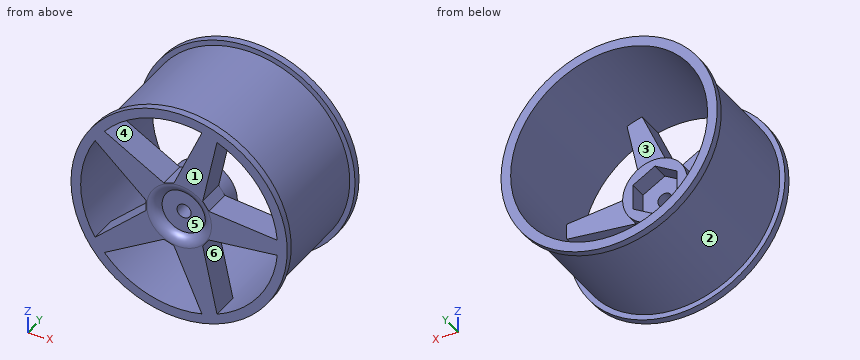
Autodesk Inventor part; units mm, degrees
ref_plane "YZ Plane" through (0, 0, 0) normal (1, 0, 0) x (0, 1, 0)
ref_plane "XZ Plane" through (0, 0, 0) normal (0, 1, 0) x (-1, 0, 0)
ref_plane "XY Plane" through (0, 0, 0) normal (0, 0, 1) x (1, 0, 0)
sketch "Sketch4" plane through (0, 0, 0) normal (0, 1, 0) x (-1, 0, 0)
  circle A0 centre (87.8745, -116.8332) radius 29.25
  point P0 (0, 0)
  dimension "d11" = 58.5
extrude "Extrusion4" add sketch "Sketch4" along normal blind 36
sketch "Sketch6" plane through (-87.8745, 0, -116.8332) normal (0, -1, 0) x (1, 0, 0)
  circle A0 centre (0, 0) radius 30.75
  point P0 (87.8745, 116.8332)
  dimension "d20" = 61.5
extrude "Extrusion6" add sketch "Sketch6" against normal blind 2
sketch "Sketch7" plane through (-87.8745, 36, -116.8332) normal (0, 1, 0) x (1, 0, 0)
  circle A0 centre (0, 0) radius 30.75
  point P0 (87.8745, -116.8332)
  dimension "d23" = 61.5
extrude "Extrusion7" add sketch "Sketch7" against normal blind 2
sketch "Sketch5" plane through (-87.8745, 0, -116.8332) normal (0, -1, 0) x (1, 0, 0)
  circle A0 centre (0, 0) radius 28
  circle A1 centre (0, 0) radius 29.25
  point P0 (87.8745, 116.8332)
  dimension "d16" = 0
  dimension "d17" = 0
  dimension "d26" = 56
extrude "Extrusion5" cut sketch "Sketch5" against normal blind 36 contours A0
sketch "Sketch8" plane through (-87.8745, 0, -116.8332) normal (0, -1, 0) x (1, 0, 0)
  circle A0 centre (0, 0) radius 8.5
  circle A1 centre (0, 0) radius 28
  line L0 (28, 0) -> (28, 2.25)
  line L1 (28, 0) -> (28, -2.25)
  line L2 (8.5, 0) -> (8.5, 4.3)
  line L3 (8.5, 0) -> (8.5, -4.3)
  line L4 (8.5, 4.3) -> (28, 2.25)
  line L5 (8.5, -4.3) -> (28, -2.25)
  arc A2 (27.9087, -2.2596) -> (27.9087, 2.2596) centre (0, 0) ccw
  line L6 (-1.4629, 9.4128) -> (6.5126, 27.3249)
  line L7 (2.6266, 8.084) -> (-1.4629, 9.4128)
  line L8 (2.6266, 8.084) -> (6.7162, 6.7552)
  line L9 (6.7162, 6.7552) -> (10.7924, 25.9343)
  arc A3 (10.7733, 25.8445) -> (6.4752, 27.241) centre (0, 0) ccw
  line L10 (-9.4041, 1.5174) -> (-23.975, 14.6377)
  line L11 (-6.8766, 4.9962) -> (-9.4041, 1.5174)
  line L12 (-6.8766, 4.9962) -> (-4.3492, 8.4749)
  line L13 (-4.3492, 8.4749) -> (-21.33, 18.2783)
  arc A4 (-21.2504, 18.2324) -> (-23.9068, 14.5763) centre (0, 0) ccw
  line L14 (-4.3492, -8.4749) -> (-21.33, -18.2783)
  line L15 (-6.8766, -4.9962) -> (-4.3492, -8.4749)
  line L16 (-6.8766, -4.9962) -> (-9.4041, -1.5174)
  line L17 (-9.4041, -1.5174) -> (-23.975, -14.6377)
  arc A5 (-23.9068, -14.5763) -> (-21.2504, -18.2324) centre (0, 0) ccw
  line L18 (6.7162, -6.7552) -> (10.7924, -25.9343)
  line L19 (2.6266, -8.084) -> (6.7162, -6.7552)
  line L20 (2.6266, -8.084) -> (-1.4629, -9.4128)
  line L21 (-1.4629, -9.4128) -> (6.5126, -27.3249)
  arc A6 (6.4752, -27.241) -> (10.7733, -25.8445) centre (0, 0) ccw
  line L22 (-1.4629, 9.4128) -> (-4.3492, 8.4749)
  line L23 (-9.4041, 1.5174) -> (-9.4041, -1.5174)
  line L24 (-4.3492, -8.4749) -> (-1.4629, -9.4128)
  line L25 (6.7162, -6.7552) -> (8.5, -4.3)
  line L26 (8.5, 4.3) -> (6.7162, 6.7552)
  line L27 (6.7162, 6.7552) -> (-1.4629, 9.4128)
  line L28 (-4.3492, 8.4749) -> (-9.4041, 1.5174)
  line L29 (-9.4041, -1.5174) -> (-4.3492, -8.4749)
  line L30 (-1.4629, -9.4128) -> (6.7162, -6.7552)
  line L31 (8.5, -4.3) -> (8.5, 4.3)
  point P0 (87.8745, 116.8332)
  point P1 (8.6525, 26.6296)
  point P2 (-22.6525, 16.458)
  point P3 (-22.6525, -16.458)
  point P4 (8.6525, -26.6296)
  dimension "d27" = 17
  dimension "d29" = 2.25
  dimension "d30" = 2.25
  dimension "d31" = 4.3
  dimension "d32" = 4.3
  dimension "d35" = 360
extrude "Extrusion8" add sketch "Sketch8" against normal blind 8 contours A0 | L3 L25 L19 A0 | A0 L8 L26 L2 | L2 L4 A1 L5 L3 | A0 L12 L22 L7 | L7 L6 A1 L9 L8 | L20 L24 L15 A0 | L19 L18 A1 L21 L20 | A0 L16 L23 L11 | L11 L10 A1 L13 L12 | L15 L14 A1 L17 L16
sketch "Sketch9" plane through (-87.8745, 0, -116.8332) normal (0, -1, 0) x (1, 0, 0)
  circle A0 centre (0, 0) radius 6.25
  point P0 (87.8745, 116.8332)
  dimension "d39" = 12.5
extrude "Extrusion9" cut sketch "Sketch9" against normal blind 2.5
fillet "Fillet1" radius 3 1 edges at (-94.1245, 0, -116.8332)
sketch "Sketch10" plane through (-87.8745, 2.5, -116.8332) normal (0, -1, 0) x (1, 0, 0)
  circle A0 centre (0, 0) radius 2
  point P0 (87.8745, 116.8332)
  dimension "d43" = 4
extrude "Extrusion10" cut sketch "Sketch10" against normal blind 50
sketch "Sketch11" plane through (-87.8745, 8, -116.8332) normal (0, 1, 0) x (1, 0, 0)
  circle A0 centre (0, 0) radius 9.208
  circle A1 centre (0, 0) radius 2
  circle A2 centre (0, 0) radius 7.208
  circle A3 centre (0, 0) radius 9.208
  line L0 (0, 7.208) -> (6.2423, 3.604)
  line L1 (6.2423, 3.604) -> (6.2423, -3.604)
  line L2 (6.2423, -3.604) -> (0, -7.208)
  line L3 (0, -7.208) -> (-6.2423, -3.604)
  line L4 (-6.2423, -3.604) -> (-6.2423, 3.604)
  line L5 (-6.2423, 3.604) -> (0, 7.208)
  point P0 (87.8745, -116.8332)
  dimension "d46" = 2
  dimension "d47" = 0
  dimension "d48" = 0
  dimension "d49" = 0
extrude "Extrusion11" add sketch "Sketch11" along normal blind 5 contours A0 | A2 L1 | L0 A2 | A2 L2 | L5 A2 | A2 L3 | L4 A2
equation "\"d30\" = d29"
equation "\"d32\" = d31"
properties part number "koleso" material "ABS Plastic"
Design review of the part built by this model. Coordinates are the model's own, in mm. Face numbers are marked on the shaded views. A direction names the side the tool comes from. Round coordinates to 2 decimals unless told otherwise and drop trailing zeros. Write each loop counter-clockwise with the first axis right and the second up, starting at its lowest first coordinate (ties: lowest second). Pieces come first, ordered by that corner, then holes. Notation, with made-up numbers: M 83.5,-11 L 96.5,-11 A19 ccw 96.5,26 Z; hole C -5,2 d11. An arc over 180 degrees is marked long. One line per item, written item: value. Start each with the question number.
1. Take a section at B-B on x = -105. State the section outline as (y, z) points, then the cut area to 3 significant figures.
2. Take a section at A-A on y = 11. State the section outline as (x, z) points, then the cut area to 3 significant figures.
3. For the marked faces 5 and 6, list the 3-axis set-ups (+Z, -Z, +X, -X, +Y, -Y) from which the entire face can be reached by the end or side of a thin tool; tool diameter is ignored.
4. Draft analysis for pull direction Z (two halves, no side actions). For the marked faces 1, 2, 3 and 4, state which applies: pulls with the +Z half, pulls with the -Z half, needs draft (parallel to the pull), parting line crosses it, or undercut.
5. To check wall thickness, follow probe 1 along X at (y, z) = (23, -140.5); probe 2 along Z at (x, y) = (-100, 6); probe 3 along Z at (x, y) = (-111, 2.5). State the ranges of each line that lie inside material, in increasing order. Write a range as from..to.
6. Clearance check with flat-ended pins moving along their axes: P1, Ø12, axis at x = -84, z = -135.5, coming from the +Y side; P2, Ø2, axis at x = -79, z = -128.5, coming from the -Y side; P3, Ø14, axis at x = -86.5, z = -118, coming from the -Y side; P4, Ø12, axis at y = 21.5, z = -108, coming from the +X side. State where each tip first meets the part, or that it passes through.
7. Take a section at D-D on y = 6. State the section outline as (x, z) points.
8. Take a section at C-C on z = -129.5. State the section outline as (x, y) points.
Computed:
1. outline: M 0,-142.37 L 2,-142.37 L 2,-140.55 L 34,-140.55 L 34,-142.37 L 36,-142.37 L 36,-138.99 L 0,-138.99 Z; M 0,-132.68 L 8,-132.68 L 8,-125.3 L 0,-125.3 Z; M 0,-108.36 L 8,-108.36 L 8,-100.98 L 0,-100.98 Z; M 0,-94.68 L 36,-94.68 L 36,-91.29 L 34,-91.29 L 34,-93.12 L 2,-93.12 L 2,-91.29 L 0,-91.29 Z
1. area: 245 mm²
2. outline: C -87.87,-116.83 d58.5; C -87.87,-116.83 d18.42; hole C -87.87,-116.83 d56; hole M -94.12,-120.44 L -87.87,-124.04 L -81.63,-120.44 L -81.63,-113.23 L -87.87,-109.63 L -94.12,-113.23 Z
2. area: 356 mm²
3. face 5: -Y
3. face 6: +Y, -Y
4. face 1: needs draft
4. face 2: parting line crosses it
4. face 3: undercut
4. face 4: undercut
5. probe 1: x = -105.06..-102.84, -72.91..-70.69
5. probe 2: z = -143.45..-142.07, -129.8..-120.8, -112.87..-103.87, -91.59..-90.21
5. probe 3: z = -134.74..-130.71, -102.96..-98.92
6. P1: stops at y = 8
6. P2: passes through
6. P3: stops at y = 0.03
6. P4: stops at x = -58.76
7. outline: C -87.87,-116.83 d58.5; hole M -111.78,-131.41 L -97.28,-118.35 L -97.28,-115.32 L -111.78,-102.26 A28 ccw Z; hole M -109.12,-135.07 A28 ccw -81.4,-144.07 L -89.34,-126.25 L -92.22,-125.31 Z; hole M -109.12,-98.6 L -92.22,-108.36 L -89.34,-107.42 L -81.4,-89.59 A28 ccw Z; hole C -87.87,-116.83 d4; hole M -81.16,-123.59 L -77.1,-142.68 A28 ccw -59.97,-119.09 L -79.37,-121.13 Z; hole M -81.16,-110.08 L -79.37,-112.53 L -59.97,-114.57 A28 ccw -77.1,-90.99 Z
8. outline: M -115.89,0 L -112.85,0 L -112.85,36 L -115.89,36 L -115.89,34 L -114.24,34 L -114.24,2 L -115.89,2 Z; M -109.66,0 L -99.48,0 L -99.48,8 L -109.66,8 Z; M -87.89,0 L -79.9,0 L -79.9,8 L -87.89,8 Z; M -62.9,0 L -59.85,0 L -59.85,2 L -61.51,2 L -61.51,34 L -59.85,34 L -59.85,36 L -62.9,36 Z
